```python
from build123d import *

# Parameters (mm, degrees)
F0_R     = 19.05
F1_DEPTH = 6
F2_R     = 12.25
F3_DEPTH = 6
F4_R     = 15.25
F5_DEPTH = 2.9
F6_SIZE  = 2


# Not quite as in the source:
# - a feature names something its author has since deleted; it is built from what else it names


with BuildPart() as f1:
    # F0 (on Top) → F1 (new body)
    with BuildSketch(Plane.XY):
        Circle(F0_R)
    extrude(amount=F1_DEPTH)

    # F2 (on face) → F3 (cut)
    with BuildSketch(Plane.XY.offset(6)):
        Circle(F2_R)
    extrude(amount=-F3_DEPTH, mode=Mode.SUBTRACT)

    # F4 (on face) → F5 (cut)
    with BuildSketch(Plane.XY.offset(6)):
        Circle(F4_R)
    extrude(amount=-F5_DEPTH, mode=Mode.SUBTRACT)

    # F6
    f6_edges = [f1.edges().sort_by_distance(p)[0] for p in [
        (-12.25, 0, 3.1),
    ]]
    chamfer(f6_edges, length=F6_SIZE)


solid = f1.part
```
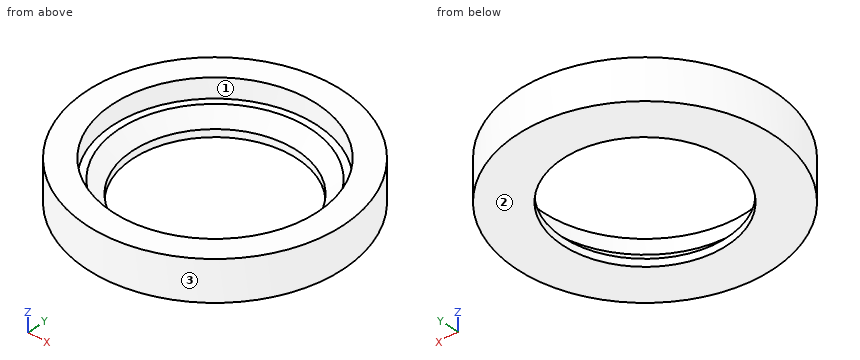
Here's how the part is built. I have some questions about the finished solid (model axes, mm). Face numbers are marked on the shaded views. Round coordinates to 2 decimals unless told otherwise and drop trailing zeros. Loops run counter-clockwise (first coordinate to the right, second up) from the corner with the lowest first, then second, coordinate; pieces in that order, holes last. Notation, with made-up numbers: (44.5, -4) -> (63.5, -4) arc R18 cw to (63.5, 9) -> close; hole circle Ø10 at (31.25, 33.5). An arc over 180 degrees is marked (long way). Answer as CSV lines item,"result". Start each with the question number.
1. If we mould it in two halves opening along Y, with no side actions, what happens to the marked faces 1, 2 and 3? For each: pulls with the +Y half, pulls with the -Y half, needs draft (parallel to the pull), parting line crosses it, or undercut.
2. Imagine slicing it at A-A on y = 0. Write out the boundary of the cut face in (x, z).
3. Imagine slicing it at D-D on z = 0.5. Write out the boundary of the cut face in (x, y).
4. Imagine slicing it at C-C on z = 5. Write out the boundary of the cut face in (x, y), plus the area to 3 significant figures.
5. I'm going to push flat-ended pins straight in: P1, Ø1.5, axis at y = -4.5, z = 1.5, coming from the +X side; P2, Ø9, axis at x = 7, y = -7, coming from the +Z side; P3, Ø4, axis at x = -2.5, y = 13.5, coming from the -Z side; P4, Ø3, axis at y = 9, z = 3, coming from the +X side. Where does each tip first touch, or does it pass through?
6. I need wall thicknesses on probe 1 along Y at (x, z) = (0, 4.25); probe 2 along Y at (x, z) = (0, 0.6); probe 3 along Z at (x, y) = (12.5, -7.5). Which ranges of each line are inside material? Lowest first, please. Write a range as from..to.
Solution:
1,face 1,"undercut"
1,face 2,"needs draft"
1,face 3,"parting line crosses it"
2,outline,"(-19.05, 0) -> (-12.25, 0) -> (-12.25, 1.1) -> (-14.25, 3.1) -> (-15.25, 3.1) -> (-15.25, 6) -> (-19.05, 6) -> close; (12.25, 0) -> (19.05, 0) -> (19.05, 6) -> (15.25, 6) -> (15.25, 3.1) -> (14.25, 3.1) -> (12.25, 1.1) -> close"
3,outline,"circle Ø38.1 at (0, 0); hole circle Ø24.5 at (0, 0)"
4,outline,"circle Ø38.1 at (0, 0); hole circle Ø30.5 at (0, 0)"
4,area,"409 mm²"
5,P1,"x = 18.68"
5,P2,"z = 3.1"
5,P3,"z = 0"
5,P4,"x = 17.51"
6,probe 1,"-19.05..-15.25, 15.25..19.05"
6,probe 2,"-19.05..-12.25, 12.25..19.05"
6,probe 3,"0..3.1"
